from build123d import *

# Parameters (mm, degrees)
F1_DEPTH = 0.889
F2_DEPTH = 1.524


with BuildPart() as f1:
    # F0 (on Front) → F1 (new body, symmetric)
    with BuildSketch(Plane.XZ):
        with BuildLine():
            Line((1.327608, -27.277179), (1.816115, -5.952824))
            Line((1.816115, -5.952824), (-2.623277, -5.952824))
            Line((-2.623277, -5.952824), (-2.623277, -27.277179))
            ThreePointArc((-2.623277, -27.277179), (-0.647834, -29.252622), (1.327608, -27.277179))
        make_face()
    extrude(amount=F1_DEPTH, both=True)

    # F0 (on Front) → F2 (join, symmetric)
    with BuildSketch(Plane.XZ):
        with BuildLine():
            Line((-2.623277, -5.952824), (1.816115, -5.952824))
            Line((1.816115, -5.952824), (4.033533, -5.952824))
            Line((4.033533, -5.952824), (6.996475, -5.952824))
            Line((6.996475, -5.952824), (8.907864, -3.839395))
            Line((8.907864, -3.839395), (8.099831, -3.165916))
            Line((8.099831, -3.165916), (5.540981, -1.507046))
            Line((5.540981, -1.507046), (2.552063, -1.507046))
            Line((2.552063, -1.507046), (-0.735558, -1.507046))
            Line((-0.735558, -1.507046), (-2.122533, -1.507046))
            Line((-2.122533, -1.507046), (-3.079158, -1.507046))
            Line((-3.079158, -1.507046), (-3.793383, -1.473681))
            ThreePointArc((-3.793383, -1.473681), (-4.641575, -3.707847), (-3.955338, -5.996954))
            Line((-3.955338, -5.996954), (-2.623277, -5.952824))
        make_face()
    extrude(amount=F2_DEPTH, both=True)


solid = f1.part
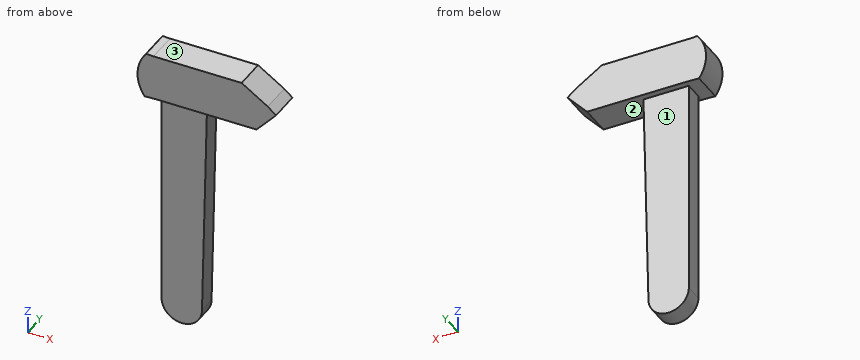
Design review of the part built by this model. Coordinates are the model's own, in mm. Face numbers are marked on the shaded views. A direction names the side the tool comes from. Give positions to 0.01 mm unless a question says otherwise; leave off trailing zeros. Write each loop counter-clockwise with the first axis right and the second up, starting at its lowest first coordinate (ties: lowest second). Pieces come first, ordered by that corner, then holes. Notation, with made-up numbers: M 17.5,19.25 L 71.5,19.25 A11 ccw 71.5,24.25 Z; hole C 88,28.5 d5. An arc over 180 degrees is marked long. Answer as a JSON object with one key per item and string values. Group by question number.
1) We need section B-B (x = 4.25). Give the boundary of the cut face in (y, z).
2) Clearance check with flat-ended pins moving along their axes: pin 1 Ø1.5 at (x, y) = (3.5, 0) entering from -Z; pin 2 Ø3.5 at (x, z) = (-0.5, -16) entering from -Y; pin 3 Ø2 at (x, z) = (0, -13) entering from +Y. State where each tip first meets the part, or that it passes through.
3) We need section D-D (y = 0.6). Give the boundary of the cut face in (x, z).
4) Tool access review of the marked faces 1, 2 and 3: name each direction out of +Z, -Z, +X, -X, +Y, -Y from which nothing blocks a thin tool from reaching the whole face with its end or side.
5) We need section A-A (y = -1.15). Give the boundary of the cut face in (x, z).
6) We need section C-C (z = -14). Give the boundary of the cut face in (x, y), and give its area (3 significant figures).
7) For line 1 along Y through (x, z) = (-1, -24); line 2 along Z through (x, y) = (1.5, 1.15); line 3 along Z through (x, y) = (1, -0.75), list the stretches that pass through material, from the lowest coordinate up.
Answer key:
{
 "1": {"outline": "M -1.52,-5.95 L 1.52,-5.95 L 1.52,-1.51 L -1.52,-1.51 Z"},
 "2": {"pin 1": "stops at z = -5.95", "pin 2": "stops at y = -0.89", "pin 3": "stops at y = 0.89"},
 "3": {"outline": "M -3.96,-6 L -2.62,-5.95 L -2.62,-27.28 A1.98 ccw 1.33,-27.28 L 1.82,-5.95 L 7,-5.95 L 8.91,-3.84 L 8.1,-3.17 L 5.54,-1.51 L -3.08,-1.51 L -3.79,-1.47 A3.72 ccw Z"},
 "4": {"face 1": "-Z, +X, -X, +Y", "face 2": "-Z, +X", "face 3": "+Z, +X, +Y, -Y"},
 "5": {"outline": "M -3.96,-6 L -2.62,-5.95 L 7,-5.95 L 8.91,-3.84 L 8.1,-3.17 L 5.54,-1.51 L -3.08,-1.51 L -3.79,-1.47 A3.72 ccw Z"},
 "6": {"outline": "M -2.62,-0.89 L 1.63,-0.89 L 1.63,0.89 L -2.62,0.89 Z", "area": "7.57 mm²"},
 "7": {"line 1": "y = -0.89 to 0.89", "line 2": "z = -5.95 to -1.51", "line 3": "z = -28.37 to -1.51"}
}
